Source: CAD feature listing. Evaluate the final solid. Frame: model axes, mm. Face numbers are marked on the shaded views. A direction names the side the tool comes from. Coordinates: 2 decimals unless noted, no trailing zeros. Write each loop counter-clockwise with the first axis right and the second up, starting at its lowest first coordinate (ties: lowest second). Pieces come first, ordered by that corner, then holes. Notation, with made-up numbers: (80.25, -25) - (95.25, -25) arc R8 ccw to (95.25, -16) - close; hole circle Ø9 at (-17.5, 19.5). An arc over 180 degrees is marked (long way). One line per item, written item: value.
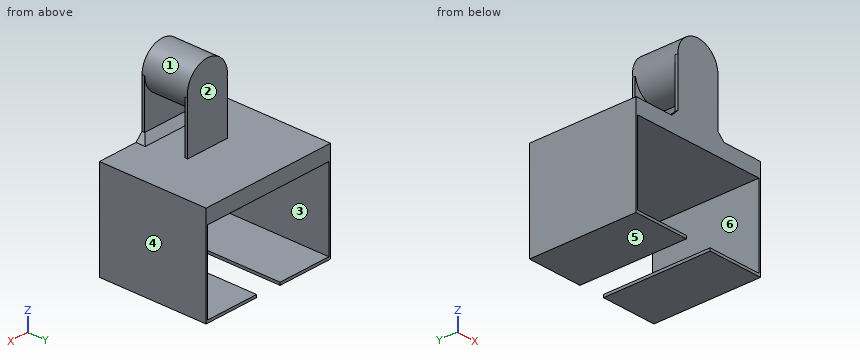
from build123d import *

# Parameters (mm, degrees)
BOSS_EXTRUDE1_DEPTH = 50.8
SKETCH3_W           = 20.832647018
SKETCH3_H           = 1.27
BOSS_EXTRUDE2_DEPTH = 25.908
SKETCH5_R           = 10.416323509
BOSS_EXTRUDE3_DEPTH = 21.59
SKETCH14_W          = 20.707274924
SKETCH14_H          = 24.296753771
BOSS_EXTRUDE7_DEPTH = 1.27
CHAMFER2_SIZE       = 3.175


with BuildPart() as part:
    # Sketch2 → Boss-Extrude1 (new body)
    with BuildSketch(Plane(origin=(0, 0, 0), x_dir=(1, 0, 0), z_dir=(0, 1, 0))):
        Polygon((66.696577012, 107.222916401), (66.696577012, 105.952916401), (41.286417012, 105.952916401), (41.286417012, 67.871966401), (104.329217012, 67.871966401), (104.329217012, 105.952916401), (78.919057012, 105.952916401), (78.919057012, 107.222916401), (105.192817012, 107.222916401), (105.192817012, 60.886966401), (40.422817012, 60.886966401), (40.422817012, 107.222916401), align=None)
    extrude(amount=BOSS_EXTRUDE1_DEPTH)

    # Sketch3 → Boss-Extrude2 (add)
    with BuildSketch(Plane.XY.offset(-60.886966401)):
        with Locations((72.594457012, 0.635)):
            Rectangle(SKETCH3_W, SKETCH3_H)
    extrude(amount=BOSS_EXTRUDE2_DEPTH)

    # Sketch5 → Boss-Extrude3 (add)
    with BuildSketch(Plane.XZ):
        with Locations(Location((72.594457012, -34.978966401, 0), (0, 0, 270))):
            Circle(SKETCH5_R)
    extrude(amount=-BOSS_EXTRUDE3_DEPTH)

    # Sketch14 → Boss-Extrude7 (add)
    with BuildSketch(Plane(origin=(0, 21.59, 0), x_dir=(1, 0, 0), z_dir=(0, 1, 0))):
        with Locations((72.531770965, 48.738589516)):
            Rectangle(SKETCH14_W, SKETCH14_H)
    extrude(amount=-BOSS_EXTRUDE7_DEPTH)

    # Chamfer2
    chamfer2_edges = [part.edges().sort_by_distance(p)[0] for p in [
        (62.178133503, 0.635, -60.886966401),
        (83.010780521, 0.635, -60.886966401),
        (72.594457012, 1.27, -60.886966401),
    ]]
    chamfer(chamfer2_edges, length=CHAMFER2_SIZE)


solid = part.part
1) Section query D-D on y = 11.5. Output: boundary loops of the cut face in (x, z).
Values found:
outline: (40.42, -107.22) - (66.7, -107.22) - (66.7, -105.95) - (41.29, -105.95) - (41.29, -67.87) - (104.33, -67.87) - (104.33, -105.95) - (78.92, -105.95) - (78.92, -107.22) - (105.19, -107.22) - (105.19, -60.89) - (40.42, -60.89) - close; circle Ø20.83 at (72.59, -34.98)
2) Reachability of the marked faces 5 and 6 from +Z, -Z, +X, -X, +Y, -Y: full face, straight path, thin tool, end or side. Return the list, or none.
Values found:
face 5: -Z, +X, -X, +Y, -Y
face 6: +Y, -Y
3) Section query B-B on x = 49. Output: boundary loops of the cut face in (y, z).
Values found:
outline: (0, -107.22) - (50.8, -107.22) - (50.8, -105.95) - (0, -105.95) - close; (0, -67.87) - (50.8, -67.87) - (50.8, -60.89) - (0, -60.89) - close
4) Section query A-A on z = -51. Output: boundary loops of the cut face in (x, y).
Values found:
outline: (62.18, 0) - (83.01, 0) - (83.01, 1.27) - (62.18, 1.27) - close; (62.18, 20.32) - (82.89, 20.32) - (82.89, 21.59) - (62.18, 21.59) - close
5) Draft query along X for the marked faces 1, 2, 3 and 4. Return one class per face: released by +X, released by -X, zero draft, split by the parting line, or undercut.
Values found:
face 1: split by the parting line
face 2: zero draft
face 3: undercut
face 4: released by +X
6) Contact query for flat-ended pins moving along their axis: P1, Ø10, axis at x = 98.5, z = -90.5, coming from the -Y side; P2, Ø10.5, axis at x = 72.5, z = -53, coming from the -Y side; P3, Ø20.5, axis at x = 91.5, y = 33, coming from the +Z side; P4, Ø10.5, axis at x = 70.5, z = -44.5, coming from the +Y side. Output: stop coordinate, or through.
Values found:
P1: through
P2: y = 0
P3: z = -60.89
P4: y = 21.59
7) Section query C-C on x = 77. Output: boundary loops of the cut face in (y, z) (3 decimals), then the cut area to 3 significant figures.
Values found:
outline: (0, -67.872) - (50.8, -67.872) - (50.8, -60.887) - (21.59, -60.887) - (21.59, -25.54) - (0, -25.54) - close; hole (1.27, -57.712) - (4.445, -60.887) - (20.32, -60.887) - (20.32, -44.418) - (1.27, -44.418) - close
area: 809 mm2
8) Material intervals for line 1 (Z direction, x = 66.5, y = 44.5); line 2 (X direction, y = 42.5, z = -86); line 3 (Y direction, x = 65.5, z = -39.5), sorted ascending.
Values found:
line 1: -107.22 to -105.95, -67.87 to -60.89
line 2: 40.42 to 41.29, 104.33 to 105.19
line 3: 0 to 21.59
